Could you check a few things on this model? Use its own coordinates, in mm. A direction names the side the tool comes from. Coordinates: 2 decimals unless noted, no trailing zeros. Order: outer loops, then holes, each group sorted by start corner. A loop starts at its lowest first (then second) coordinate and runs counter-clockwise, first axis right, second up. Notation, with made-up numbers: (-2.5, -1) - (19.5, -1) arc R29 cw to (19.5, 27) - close; hole circle Ø10 at (51, 77.25). An arc over 180 degrees is marked (long way). Answer as a JSON object with one key per item and string values. Group by question number.
(1) Imagine slicing it at C-C, the plane y = 0.75. Write out the boundary of the cut face in (x, z).
(2) We'd pull the mould along Z, two halves only. Please class faces 1 (the flat face through (-5, -5.4, 0.1)), 2 (the cylindrical face through (7.32, 7.43, -9.4)), 3 (the flat face through (7, 0, 7.56)): pulls with the +Z half, pulls with the -Z half, needs draft (parallel to the pull), parting line crosses it, or undercut.
(3) Imagine slicing it at A-A, the plane z = 0. Write out the boundary of the cut face in (x, y).
(4) Please list where these lines run through material, in increasing order: probe 1 along Y at (x, z) = (-2, -5); probe 2 along Z at (x, y) = (0, -6.4); probe 3 along X at (y, z) = (-6.9, 0).
(5) Imagine slicing it at B-B, the plane x = 5. Write out the boundary of the cut face in (y, z), and give its area (3 significant figures).
(6) Which directions (+Z, -Z, +X, -X, +Y, -Y) give clear straight access to the entire face, cutting with the end or side of a thin tool? Please do faces 4 (the flat face through (8, -1, 10)), 5 (the flat face through (7, 0, -7.56)).
(7) Imagine slicing it at D-D, the plane y = 6.5. Write out the boundary of the cut face in (x, z), and give its area (3 significant figures).
(8) Will these pins go through, and if not, where does the flat tip stop? P1, Ø1.9, axis at x = 0, z = 0, coming from the -Y side; P2, Ø2, axis at x = 26.5, y = 5.5, coming from the +Z side; P3, Ø5, axis at y = -1.5, z = 2.5, coming from the -X side; P4, Ø2, axis at x = 0.5, z = 1, coming from the -Y side.
Autodesk Inventor part; units mm, degrees
ref_plane "YZ Plane" through (0, 0, 0) normal (1, 0, 0) x (0, 1, 0)
ref_plane "XZ Plane" through (0, 0, 0) normal (0, 1, 0) x (-1, 0, 0)
ref_plane "XY Plane" through (0, 0, 0) normal (0, 0, 1) x (1, 0, 0)
sketch "Sketch1" plane through (0, 0, 0) normal (0, 1, 0) x (-1, 0, 0)
  line L0 (5, -10) -> (-20, -10)
  line L1 (-20, -10) -> (-20, 10)
  line L2 (-20, 10) -> (5, 10)
  line L3 (5, 10) -> (5, -10)
  line L4 (5, -10) -> (-20, 10) construction
  line L5 (-20, -10) -> (5, 10) construction
  circle A0 centre (-20, 0) radius 10
  point P0 (0, 0)
  point P1 (-7.5, 0)
  point P2 (-20, 10)
  dimension "d0" = 20
  dimension "d1" = 20
  dimension "d2" = 5
extrude "Extrusion1" add sketch "Sketch1" along normal mid plane 16
sketch "Sketch2" plane through (0, 8, 0) normal (0, 1, 0) x (1, 0, 0)
  point P0 (0, 0)
  point P1 (0, 0)
hole "Hole1" at (0, 8, 0) direction (0, -1, 0) diameter 3.1 end through all
sketch "Sketch3" plane through (-5, -8, 10) normal (-1, 0, 0) x (0, 0, 1)
  line L0 (-17.56, 2.94) -> (-2.44, 2.94)
  line L1 (-2.44, 2.94) -> (-2.44, 13.06)
  line L2 (-2.44, 13.06) -> (-17.56, 13.06)
  line L3 (-17.56, 13.06) -> (-17.56, 2.94)
  line L4 (-17.56, 2.94) -> (-2.44, 13.06) construction
  line L5 (-2.44, 2.94) -> (-17.56, 13.06) construction
  point P0 (-10, 8)
  dimension "d12" = 15.12
  dimension "d13" = 10.12
extrude "Extrusion2" cut sketch "Sketch3" against normal blind 24.5
fillet "Fillet1" radius 2 3 edges at (30, 8, 0) (7.5, 8, -10) (7.5, 8, 10)
properties part number "T-Frame Left Cover" material "ABS Plastic"
Result set:
{
 "1": {"outline": "(-5, -10) - (20, -10) arc R10 ccw to (20, 10) - (-5, 10) - (-5, 7.56) - (19.5, 7.56) - (19.5, -7.56) - (-5, -7.56) - close"},
 "2": {"face 1": "needs draft", "face 2": "pulls with the -Z half", "face 3": "undercut"},
 "3": {"outline": "(-5, -8) - (-1.55, -8) - (-1.55, -5.06) - (-5, -5.06) - close; (-5, 5.06) - (-1.55, 5.06) - (-1.55, 8) - (-5, 8) - close; (1.55, -8) - (30, -8) - (30, 6) arc R2 ccw to (28, 8) - (1.55, 8) - (1.55, 5.06) - (19.5, 5.06) - (19.5, -5.06) - (1.55, -5.06) - close"},
 "4": {"probe 1": "y = -8 to -5.06, 5.06 to 8", "probe 2": "z = -10 to -1.55, 1.55 to 10", "probe 3": "x = -5 to -1.55, 1.55 to 30"},
 "5": {"outline": "(-8, -10) - (6, -10) arc R2 ccw to (8, -8) - (8, 8) arc R2 ccw to (6, 10) - (-8, 10) - close; hole (-5.06, -7.56) - (5.06, -7.56) - (5.06, 7.56) - (-5.06, 7.56) - close", "area": "165 mm^2"},
 "6": {"face 4": "+Z, +X, -X, +Y, -Y", "face 5": "-X"},
 "7": {"outline": "(-5, -9.94) - (20, -9.94) arc R9.94 ccw to (20, 9.94) - (-5, 9.94) - close; hole circle Ø3.1 at (0, 0)", "area": "644 mm^2"},
 "8": {"P1": "passes through", "P2": "stops at z = 8.35", "P3": "stops at x = 19.5", "P4": "stops at y = -8"}
}
